Can you work these out from the model? Positions are in its coordinate system, mm. Give positions to 0.01 mm unless a question says otherwise; leave off trailing zeros. Answer as a JSON object with one key per item and string values.
Autodesk Inventor part; units mm, degrees
ref_plane "YZ Plane" through (0, 0, 0) normal (1, 0, 0) x (0, 1, 0)
ref_plane "XZ Plane" through (0, 0, 0) normal (0, 1, 0) x (-1, 0, 0)
ref_plane "XY Plane" through (0, 0, 0) normal (0, 0, 1) x (1, 0, 0)
sketch "Sketch1" plane through (0, 0, 0) normal (1, 0, 0) x (0, 1, 0)
  line L0 (0, 0) -> (10, 0)
  line L1 (10, 0) -> (10, -18)
  line L2 (10, -18) -> (0, -18)
  line L3 (0, -18) -> (0, 0)
  spline S0 degree 4 poles (3.4811, -17.7286) (4.0754, -16.5984) (6.7935, -13.1301) (4.9927, -3.6489) (3.9933, 0.2842) (2.722, 0) knots 0 0 0 0 0 0.526556 1 1 1 1 1
  spline S1 degree 3 poles (2.722, 0) (1.0371, -0.5817) (5.854, -12.0092) (3.4811, -17.7286) knots 0 0 0 0 1 1 1 1
  point P0 (4.392, -16.0283)
  point P1 (5.4548, -11.4431)
  point P2 (4.8476, -3.8821)
  point P3 (3.6937, -0.39)
  point P4 (2.3577, -0.8758)
  point P5 (3.4812, -7.5865)
  dimension "d0" = 10
  dimension "d1" = 18
extrude "Extrusion1" add sketch "Sketch1" along normal blind 36 contours S0 L0 | L0 S0 S1
sketch "Sketch2" plane through (36, 0, 0) normal (1, 0, 0) x (0, 0, -1)
  line L0 (4.2519, 4) -> (9.2519, 4)
  line L1 (9.2519, 4) -> (9.2519, 0)
  line L2 (9.2519, 0) -> (4.2519, 0)
  line L3 (4.2519, 0) -> (4.2519, 4)
  point P0 (0, 0)
  dimension "d4" = 5
  dimension "d7" = 4
extrude "Extrusion2" add sketch "Sketch2" against normal blind 4
mirror "Mirror1" about plane through (36, 4.1406, -8.6966) normal (1, 0, 0)
sketch "Sketch3" plane through (32, 0, -9.2519) normal (0, -1, 0) x (1, 0, 0)
  line L0 (0, 5) -> (8, 5)
  line L1 (8, 5) -> (8, 0)
  line L2 (8, 0) -> (0, 0)
  line L3 (0, 0) -> (0, 5)
  point P0 (-32, 9.2519)
extrude "Extrusion3" add sketch "Sketch3" along normal blind 2
fillet "Fillet1" radius 2.5 1 edges at (40, 0.4133, -4.2519)
fillet "Fillet2" radius 2.5 1 edges at (32, 0.4133, -4.2519)
fillet "Fillet3" radius 2.5 1 edges at (40, 0.8821, -9.2519)
fillet "Fillet4" radius 2.5 1 edges at (32, 0.8821, -9.2519)
properties part number "2015 Back Spoiler 1"
1) I'm going to push flat-ended pins straight in: pin 1 Ø0.9 at (x, y) = (36, 1) entering from +Z; pin 2 Ø8 at (x, z) = (22, -13.5) entering from -Y; pin 3 Ø8 at (x, z) = (11, -4.5) entering from -Y. Where does each tip first touch, or does it pass through?
Results found:
{"pin 1": "stops at z = -4.25", "pin 2": "stops at y = 3.57", "pin 3": "stops at y = 2.36"}
2) I need wall thicknesses on L1, parallel to Z at x = 35.5, y = 3; L2, parallel to Y at x = 60, z = -1.25; L3, parallel to Y at x = 18, z = -8.75. Which ranges of each line are inside material? Lowest first, please.
Results found:
{"L1": "z = -9.25 to 0.02", "L2": "y = 2.36 to 4.16", "L3": "y = 3.68 to 5.45"}
3) Thinking about a two-plate mould opening in X: for faces 1 (the face through (39.248, 0.699, -4.965)), 2 (the face through (36, 0, -4.252)), 3 (the face through (32.752, 0.625, -4.965)), which applies, pulls with the +X half, pulls with the -X half, needs draft (parallel to the pull), parting line crosses it, or undercut?
Results found:
{"face 1": "pulls with the +X half", "face 2": "needs draft", "face 3": "pulls with the -X half"}
